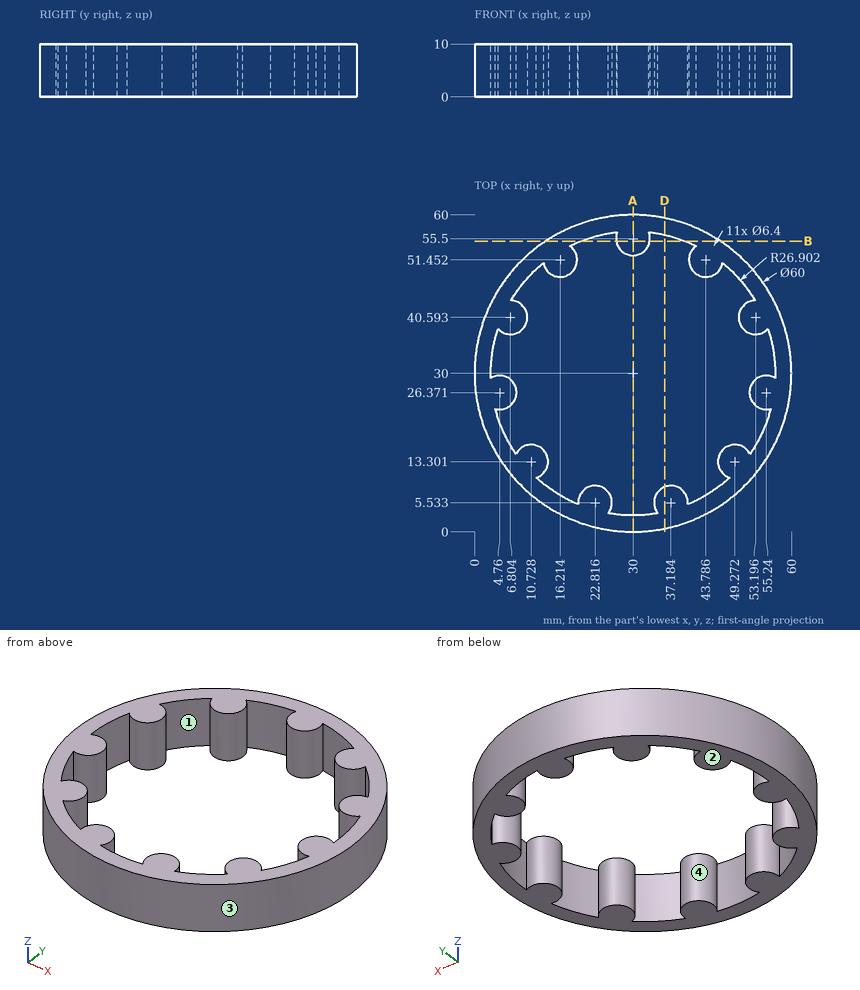
Geometry: see drawing. Coordinates: mm, zero at the bounding-box minimum. Give positions to 0.01 mm unless a question says otherwise; leave off trailing zeros. Order: outer loops, then holes, each group sorted by start corner. A loop starts at its lowest first (then second) coordinate and runs counter-clockwise, first axis right, second up.
Q1. Section D-D on x = 36. Output: boundary loops of the cut face in (y, z) (1 decimal), and give its area (3 significant figures).
Checked values:
outline: (0.6, 0) - (8.5, 0) - (8.5, 10) - (0.6, 10) - close; (56.2, 0) - (59.4, 0) - (59.4, 10) - (56.2, 10) - close
area: 111 mm2
Q2. Draft query along Y for the marked faces 1, 2, 3 and 4. Return one class per face: +Y half, -Y half, draft (parallel to the pull), parting line (faces both ways), or undercut.
Checked values:
face 1: undercut
face 2: draft
face 3: parting line
face 4: undercut
Q3. Ray query, probe 1 along Y at (x, z) = (30, 1.5); probe 2 along X at (y, z) = (5.5, 6.5) (1 decimal); probe 3 along X at (y, z) = (54.5, 7.5) (1 decimal). Return the intervals inside material, ascending.
Checked values:
probe 1: y = 0 to 3.1, 52.3 to 60
probe 2: x = 12.7 to 18.9, 19.6 to 26, 34 to 40.4, 41.1 to 47.3
probe 3: x = 12.7 to 18.9, 27 to 33, 41.1 to 47.3
Q4. Section A-A on x = 30. Output: boundary loops of the cut face in (y, z).
Checked values:
outline: (0, 0) - (3.1, 0) - (3.1, 10) - (0, 10) - close; (52.3, 0) - (60, 0) - (60, 10) - (52.3, 10) - close
Q5. Contact query for flat-ended pins moving along their axis: pin 1 Ø3 at (y, z) = (45.5, 9) entering from -X; pin 2 Ø6 at (y, z) = (39, 5.5) entering from +X; pin 3 Ø1.5 at (x, z) = (44.5, 7) entering from -Y. Output: stop coordinate, or through.
Checked values:
pin 1: stops at x = 3.47
pin 2: stops at x = 59.39
pin 3: stops at y = 3.34
Q6. Section B-B on y = 55. Output: boundary loops of the cut face in (x, z) (1 decimal).
Checked values:
outline: (13.4, 0) - (20.1, 0) - (20.1, 10) - (13.4, 10) - close; (26.8, 0) - (33.2, 0) - (33.2, 10) - (26.8, 10) - close; (39.9, 0) - (46.6, 0) - (46.6, 10) - (39.9, 10) - close
